Check sheet for the modelled part. Datum: model origin and axes. Units: mm. A direction names the side the tool comes from. Give positions to 0.01 mm unless a question says otherwise; leave off trailing zeros. Write each loop counter-clockwise with the first axis right and the second up, starting at its lowest first coordinate (ties: lowest second). Pieces come first, ordered by that corner, then holes. Notation, with made-up numbers: (68.25, 4.5) -> (74.25, 4.5) arc R18 ccw to (74.25, 11.5) -> close; hole circle Ø4 at (53, 89). An arc over 180 degrees is marked (long way). Answer as a JSON object with one key per item and string values.
Autodesk Inventor part; units mm, degrees
ref_plane "YZ Plane" through (0, 0, 0) normal (1, 0, 0) x (0, 1, 0)
ref_plane "XZ Plane" through (0, 0, 0) normal (0, 1, 0) x (-1, 0, 0)
ref_plane "XY Plane" through (0, 0, 0) normal (0, 0, 1) x (1, 0, 0)
sketch "Sketch1" plane through (0, 0, 0) normal (0, 0, 1) x (1, 0, 0)
  line L0 (0, 0) -> (-24, 0)
  line L1 (-24, 0) -> (-24, 23)
  line L2 (-24, 23) -> (0, 23)
  line L3 (0, 23) -> (0, 0)
  line L4 (-24, 17.8038) -> (-19, 17.8038)
  line L5 (-19, 17.8038) -> (-16, 23)
  dimension "d0" = 23
  dimension "d1" = 24
  dimension "d2" = 120
  dimension "d3" = 5
  dimension "d4" = 6
extrude "Extrusion1" add sketch "Sketch1" along normal blind 6.5 contours L0 L1 L4 L5 L2 L3
properties part number "Cam_SD_base"
1. Go/stop test with a flat-tipped pin: P1, Ø2, axis at y = 18.5, z = 3, coming from the -X side. Record where the tip stops, or that it passes through.
Determined:
{"P1": "x = -24"}
2. Scan lines: L1, parallel to Y at x = -20.5, z = 3; L2, parallel to Y at x = -18, z = 2.5. Record each from-to range of solid material in increasing order. Write a range as [from, to].
Determined:
{"L1": "[0, 17.8]", "L2": "[0, 19.54]"}
3. Sectioned sample at A-A, the plane z = 0.5. Enter the section's corners in (x, y), plus the area to 3 significant figures.
Determined:
{"outline": "(-24, 0) -> (0, 0) -> (0, 23) -> (-16, 23) -> (-19, 17.8) -> (-24, 17.8) -> close", "area": "518 mm^2"}
4. Sectioned sample at C-C, the plane y = 20.75. Enter the section's corners in (x, z).
Determined:
{"outline": "(-17.3, 0) -> (0, 0) -> (0, 6.5) -> (-17.3, 6.5) -> close"}
5. Access from +Z, -Z, +X, -X, +Y, -Y to the whole of each face (thin tool, end or side, straight path). Record for faces 1 (the face through (-22, 17.804, 3)), 2 (the face through (0, 12, 3)).
Determined:
{"face 1": "+Z, -Z, -X, +Y", "face 2": "+Z, -Z, +X, +Y, -Y"}
6. Sectioned sample at B-B, the plane x = -20. Enter the section's corners in (y, z).
Determined:
{"outline": "(0, 0) -> (17.8, 0) -> (17.8, 6.5) -> (0, 6.5) -> close"}
